```python
from build123d import *

# Parameters (mm, degrees)
SKETCH1_R               = 22.225
SKETCH1_R_2             = 18.415
BOSS_EXTRUDE1_DEPTH     = 33.02
CUT_EXTRUDE1_DEPTH      = 43.18
CUT_EXTRUDE1_DEPTH_BACK = 43.18
SKETCH2_R               = 1.4224
CUT_EXTRUDE2_DEPTH      = 43.18
CUT_EXTRUDE2_DEPTH_BACK = 43.18
SKETCH3_R               = 1.4224
SKETCH4_W               = 49.025527768
SKETCH4_H               = 48.000320082
SKETCH4_W_2             = 44.069
SKETCH4_H_2             = 44.069
CUT_EXTRUDE3_DEPTH      = 19.177
BOSS_EXTRUDE2_START     = -4.826
SKETCH5_R               = 24.765
SKETCH5_R_2             = 18.415
BOSS_EXTRUDE2_DEPTH     = 4.826


with BuildPart() as part:
    # Sketch1 → Boss-Extrude1 (new body)
    with BuildSketch(Plane(origin=(0, 0, 0), x_dir=(1, 0, 0), z_dir=(0, 1, 0))):
        with Locations(Location((0, 0, 0), (0, 0, 270))):
            Circle(SKETCH1_R)
        with Locations(Location((0, 0, 0), (0, 0, 270))):
            Circle(SKETCH1_R_2, mode=Mode.SUBTRACT)
    extrude(amount=BOSS_EXTRUDE1_DEPTH)

    # Sketch2 → Cut-Extrude1 (cut, two sides: drawn at the far end of the back side and taken through both)
    with BuildSketch(Plane.XY.offset(-CUT_EXTRUDE1_DEPTH_BACK)):
        with Locations(Location((0, 3.81, 0), (0, 0, 180))):
            Circle(SKETCH2_R)
    extrude(amount=CUT_EXTRUDE1_DEPTH + CUT_EXTRUDE1_DEPTH_BACK, mode=Mode.SUBTRACT)

    # Sketch3 → Cut-Extrude2 (cut, two sides: drawn at the far end of the back side and taken through both)
    with BuildSketch(Plane(origin=(0, 0, 0), x_dir=(0, 0, -1), z_dir=(1, 0, 0)).offset(-CUT_EXTRUDE2_DEPTH_BACK)):
        with Locations(Location((0, 3.81, 0), (0, 0, 180))):
            Circle(SKETCH3_R)
    extrude(amount=CUT_EXTRUDE2_DEPTH + CUT_EXTRUDE2_DEPTH_BACK, mode=Mode.SUBTRACT)

    # Sketch4 → Cut-Extrude3 (cut)
    with BuildSketch(Plane.XZ):
        Rectangle(SKETCH4_W, SKETCH4_H)
        Rectangle(SKETCH4_W_2, SKETCH4_H_2, mode=Mode.SUBTRACT)
    extrude(amount=-CUT_EXTRUDE3_DEPTH, mode=Mode.SUBTRACT)

    # Sketch5 → Boss-Extrude2 (add)
    with BuildSketch(Plane(origin=(0, 24.003, 0), x_dir=(1, 0, 0), z_dir=(0, 1, 0)).offset(BOSS_EXTRUDE2_START)):
        with Locations(Location((0, 0, 0), (0, 0, 270))):
            Circle(SKETCH5_R)
        with Locations(Location((0, 0, 0), (0, 0, 270))):
            Circle(SKETCH5_R_2, mode=Mode.SUBTRACT)
    extrude(amount=BOSS_EXTRUDE2_DEPTH)


solid = part.part
```
Verification items for the finished model (mm, model axes). A direction names the side the tool comes from. Coordinates: 2 decimals unless noted, no trailing zeros. Order: outer loops, then holes, each group sorted by start corner. A loop starts at its lowest first (then second) coordinate and runs counter-clockwise, first axis right, second up. Notation, with made-up numbers: (69.5, -36.5) -> (91.5, -36.5) arc R24 ccw to (91.5, 1.5) -> close; hole circle Ø2 at (47, 4). An arc over 180 degrees is marked (long way). Put each result on its own line as item: value. Start each with the question number.
1) Cross-section at A-A (x = 0). Enter the section's corners in (y, z) (1 decimal), plus the area to 3 significant figures.
2) Release check for a two-part mould opening along Y. For faces 1 (the cylindrical face through (15.57, 9.45, 15.86)), 2 (the flat face through (17, 33.02, -8)), 3 (the cylindrical face through (0.2, 2.4, 20.2)) record: pulls with the +Y half, pulls with the -Y half, needs draft (parallel to the pull), parting line crosses it, or undercut.
3) Cross-section at D-D (x = -10). Enter the section's corners in (y, z).
4) Cross-section at C-C (z = 0). Enter the section's corners in (x, y) (1 decimal).
5) Tool access check on faces 4 (the cylindrical face through (-15.57, 9.45, -15.86)), 5 (the flat face through (0, 9, 22.034)), 6 (the flat face through (15, 24.003, -17)), 7 (the flat face through (-3.6, 19.177, -22.1)), 8 (the cylindrical face through (-15.86, 9.45, 15.57)). Record the directions out of +Z, -Z, +X, -X, +Y, -Y that give a thin tool (end or side, any length) a straight path to the whole face; none if there is none.
6) Go/stop test with flat-tipped pins: pin 1 (2 mm diameter, centred on x = 3, y = 15.5, fed in from -Z); pin 2 (10 mm diameter, centred on y = 9.5, z = -9, fed in from -X); pin 3 (5 mm diameter, centred on x = 11.5, y = 20.5, fed in from +Z); pin 4 (22 mm diameter, centred on x = 0, z = 0, fed in from -Y). Record where each tip stops, or that it passes through.
7) Material ranges on L1, parallel to Y at x = 0, z = 21; L2, parallel to X at y = 24.5, z = 0 (3 decimals); L3, parallel to Z at x = -15, y = 25.5, recorded low to high.
Geometry check:
1. outline: (0, -22) -> (2.4, -22) -> (2.4, -18.4) -> (0, -18.4) -> close; (0, 18.4) -> (2.4, 18.4) -> (2.4, 22) -> (0, 22) -> close; (5.2, -22) -> (19.2, -22) -> (19.2, -24.8) -> (24, -24.8) -> (24, -22.2) -> (33, -22.2) -> (33, -18.4) -> (5.2, -18.4) -> close; (5.2, 18.4) -> (33, 18.4) -> (33, 22.2) -> (24, 22.2) -> (24, 24.8) -> (19.2, 24.8) -> (19.2, 22) -> (5.2, 22) -> close
1. area: 248 mm^2
2. face 1: needs draft
2. face 2: pulls with the +Y half
2. face 3: undercut
3. outline: (0, -19.85) -> (19.18, -19.85) -> (19.18, -22.66) -> (24, -22.66) -> (24, -19.85) -> (33.02, -19.85) -> (33.02, -15.46) -> (0, -15.46) -> close; (0, 15.46) -> (33.02, 15.46) -> (33.02, 19.85) -> (24, 19.85) -> (24, 22.66) -> (19.18, 22.66) -> (19.18, 19.85) -> (0, 19.85) -> close
4. outline: (-24.8, 19.2) -> (-22, 19.2) -> (-22, 5.2) -> (-18.4, 5.2) -> (-18.4, 33) -> (-22.2, 33) -> (-22.2, 24) -> (-24.8, 24) -> close; (-22, 0) -> (-18.4, 0) -> (-18.4, 2.4) -> (-22, 2.4) -> close; (18.4, 0) -> (22, 0) -> (22, 2.4) -> (18.4, 2.4) -> close; (18.4, 5.2) -> (22, 5.2) -> (22, 19.2) -> (24.8, 19.2) -> (24.8, 24) -> (22.2, 24) -> (22.2, 33) -> (18.4, 33) -> close
5. face 4: -Z, -X, -Y
5. face 5: +Z, +X, -X, -Y
5. face 6: +Y
5. face 7: -Y
5. face 8: +Z, -X, -Y
6. pin 1: stops at z = -22.03
6. pin 2: stops at x = -21.86
6. pin 3: stops at z = 23.07
6. pin 4: passes through
7. L1: y = 0 to 2.39, 5.23 to 33.02
7. L2: x = -22.225 to -18.415, 18.415 to 22.225
7. L3: z = -16.4 to -10.68, 10.68 to 16.4
